```python
from build123d import *

# Parameters (mm, degrees)
SKETCH1_R           = 6
SKETCH1_R_2         = 1.3
BOSS_EXTRUDE1_DEPTH = 8
SKETCH4_W           = 8
SKETCH4_H           = 3
BOSS_EXTRUDE2_DEPTH = 6
BOSS_EXTRUDE4_DEPTH = 6
SKETCH12_R          = 1.3
CUT_EXTRUDE6_DEPTH  = 6
SKETCH13_R          = 1.3
CUT_EXTRUDE7_DEPTH  = 6
SKETCH14_R          = 3
CUT_EXTRUDE8_DEPTH  = 3


with BuildPart() as part:
    # Sketch1 → Boss-Extrude1 (new body)
    with BuildSketch(Plane.XY):
        Circle(SKETCH1_R)
        Circle(SKETCH1_R_2, mode=Mode.SUBTRACT)
        with BuildLine():
            ThreePointArc((0, -6), (-4.242640687, -4.242640687), (-6, 0))
            Line((-6, 0), (-6, -6))
            Line((-6, -6), (0, -6))
        make_face()
        with BuildLine():
            Line((6, 6), (0, 6))
            ThreePointArc((0, 6), (4.242640687, 4.242640687), (6, 0))
            Line((6, 0), (6, 6))
        make_face()
    extrude(amount=BOSS_EXTRUDE1_DEPTH)

    # Sketch4 → Boss-Extrude2 (add)
    with BuildSketch(Plane(origin=(0, 0, 0), x_dir=(0, 0, -1), z_dir=(1, 0, 0))):
        with Locations((-4, -7.5)):
            Rectangle(SKETCH4_W, SKETCH4_H)
        with BuildLine():
            Line((-8, -9), (0, -9))
            ThreePointArc((0, -9), (-4, -13), (-8, -9))
        make_face()
    extrude(amount=-BOSS_EXTRUDE2_DEPTH)

    # Sketch5 → Boss-Extrude4 (add)
    with BuildSketch(Plane(origin=(0, 0, 0), x_dir=(1, 0, 0), z_dir=(0, 1, 0))):
        with BuildLine():
            Line((6, 0), (9, 0))
            ThreePointArc((9, 0), (13, -4), (9, -8))
            Line((9, -8), (6, -8))
            Line((6, -8), (6, 0))
        make_face()
    extrude(amount=BOSS_EXTRUDE4_DEPTH)

    # Sketch12 → Cut-Extrude6 (cut)
    with BuildSketch(Plane.XZ):
        with Locations((9, 4)):
            Circle(SKETCH12_R)
    extrude(amount=-CUT_EXTRUDE6_DEPTH, mode=Mode.SUBTRACT)

    # Sketch13 → Cut-Extrude7 (cut)
    with BuildSketch(Plane(origin=(0, 0, 0), x_dir=(0, 0, -1), z_dir=(1, 0, 0))):
        with Locations((-4, -9)):
            Circle(SKETCH13_R)
    extrude(amount=-CUT_EXTRUDE7_DEPTH, mode=Mode.SUBTRACT)

    # Sketch14 → Cut-Extrude8 (cut)
    with BuildSketch(Plane(origin=(0, 0, 0), x_dir=(-1, 0, 0), z_dir=(0, 0, -1))):
        Circle(SKETCH14_R)
    extrude(amount=-CUT_EXTRUDE8_DEPTH, mode=Mode.SUBTRACT)


solid = part.part
```
Could you check a few things on this model? Use its own coordinates, in mm. A direction names the side the tool comes from. Coordinates: 2 decimals unless noted, no trailing zeros. Loops run counter-clockwise (first coordinate to the right, second up) from the corner with the lowest first, then second, coordinate; pieces in that order, holes last. Notation, with made-up numbers: M 67.25,-37 L 83.25,-37 A24 cw 83.25,-3 Z; hole C -6.75,-19.75 d4. An arc over 180 degrees is marked long. Put each result on its own line as item: value. Start each with the question number.
(1) I need wall thicknesses on line 1 (Z direction, x = 9, y = 2); line 2 (X direction, y = -7.75, z = 7.75); line 3 (Z direction, x = -1.5, y = -0.5). Which ranges of each line are inside material? Lowest first, please. Write a range as from..to.
(2) For faces 1 (the face through (-1.3, 0.7, 3)), 2 (the face through (0, -10.23, 3.17)), 3 (the face through (7, 6, 4)), which set-ups out of +Z, -Z, +X, -X, +Y, -Y let a thin tool reach every point of the face, with its end or its side?
(3) Suppose I cut it at B-B on x = -2. Please give me the cut outline in (y, z).
(4) Suppose I cut it at A-A on z = 4. Please give me the cut outline in (x, y).
(5) Will these pins go through, and if not, where does the flat tip stop? P1, Ø4, axis at y = -6.5, z = 7, coming from the +X side; P2, Ø3.5, axis at x = 0, y = 0, coming from the -Z side; P3, Ø2, axis at y = -10.5, z = 4.5, coming from the +X side.
(6) Suppose I cut it at C-C on y = -0.5. Please give me the cut outline in (x, z), then the cut area to 3 significant figures.
(7) Suppose I cut it at D-D on z = 5.75. Please give me the cut outline in (x, y).
(8) Thinking about a two-plate mould opening in Z: for faces 4 (the face through (1, -3, 0)), 5 (the face through (-4.196, 4.289, 3.944)), 6 (the face through (-2.96, -7.71, 4.17)), which applies, pulls with the +Z half, pulls with the -Z half, needs draft (parallel to the pull), parting line crosses it, or undercut?
Solutions:
1. line 1: z = 0..2.7, 5.3..8
1. line 2: x = -6..0
1. line 3: z = 3..8
2. face 1: -Z
2. face 2: +Z, -Z, +X, -Y
2. face 3: +Z, -Z, +X, -X, +Y
3. outline: M -9,0 L -2.24,0 L -2.24,3 L 2.24,3 L 2.24,0 L 5.66,0 L 5.66,8 L -9,8 A4 ccw Z; hole C -9,4 d2.6
4. outline: M -6,-13 L 0,-13 L 0,-10.3 L -6,-10.3 Z; M -6,-7.7 L 0,-7.7 L 0,-6 A6 ccw 6,0 L 7.7,0 L 7.7,6 L 0,6 A6 ccw -6,0 Z; M 10.3,0 L 13,0 L 13,6 L 10.3,6 Z; hole C 0,0 d2.6
5. P1: stops at x = 3.97
5. P2: stops at z = 3
5. P3: stops at x = 0
6. outline: M -6,0 L -2.96,0 L -2.96,3 L -1.2,3 L -1.2,8 L -6,8 Z; M 1.2,3 L 2.96,3 L 2.96,0 L 5.98,0 L 5.98,8 L 1.2,8 Z
6. area: 66.1 mm2
7. outline: M -6,-12.6 L 0,-12.6 L 0,-6 A6 ccw 6,0 L 12.6,0 L 12.6,6 L 0,6 A6 ccw -6,0 Z; hole C 0,0 d2.6
8. face 4: pulls with the -Z half
8. face 5: needs draft
8. face 6: undercut
